```python
from build123d import *

# Parameters (mm, degrees)
SKETCH1_W           = 144
SKETCH1_H           = 50
SKETCH1_R           = 6
BOSS_EXTRUDE1_DEPTH = 37.5
SKETCH2_W           = 51
SKETCH2_H           = 38
CUT_EXTRUDE1_DEPTH  = 157.978501713
CUT_EXTRUDE2_DEPTH  = 116.364639296


with BuildPart() as part:
    # Sketch1 → Boss-Extrude1 (new, symmetric)
    with BuildSketch(Plane(origin=(0, 0, 0), x_dir=(0, 0, -1), z_dir=(1, 0, 0))):
        with Locations((0, 25)):
            Rectangle(SKETCH1_W, SKETCH1_H)
        with Locations((-19, 31)):
            Circle(SKETCH1_R, mode=Mode.SUBTRACT)
        with Locations(Location((19, 31, 0), (0, 0, 180))):
            Circle(SKETCH1_R, mode=Mode.SUBTRACT)
    extrude(amount=BOSS_EXTRUDE1_DEPTH, both=True)

    # Sketch2 → Cut-Extrude1 (cut, through all)
    with BuildSketch(Plane.XY.offset(72)):
        with Locations((0, 31)):
            Rectangle(SKETCH2_W, SKETCH2_H)
    extrude(amount=-CUT_EXTRUDE1_DEPTH, mode=Mode.SUBTRACT)

    # Sketch3 → Cut-Extrude2 (cut, through all)
    with BuildSketch(Plane(origin=(37.5, 0, 0), x_dir=(0, 0, -1), z_dir=(1, 0, 0))):
        with BuildLine():
            Line((72, 12), (72, 50))
            Line((72, 50), (37.5, 50))
            ThreePointArc((37.5, 50), (49.502162082, 26.235515574), (72, 12))
        make_face()
        with BuildLine():
            Line((-72, 50), (-37.5, 50))
            ThreePointArc((-37.5, 50), (-49.502162082, 26.235515574), (-72, 12))
            Line((-72, 12), (-72, 50))
        make_face()
    extrude(amount=-CUT_EXTRUDE2_DEPTH, mode=Mode.SUBTRACT)


solid = part.part
```
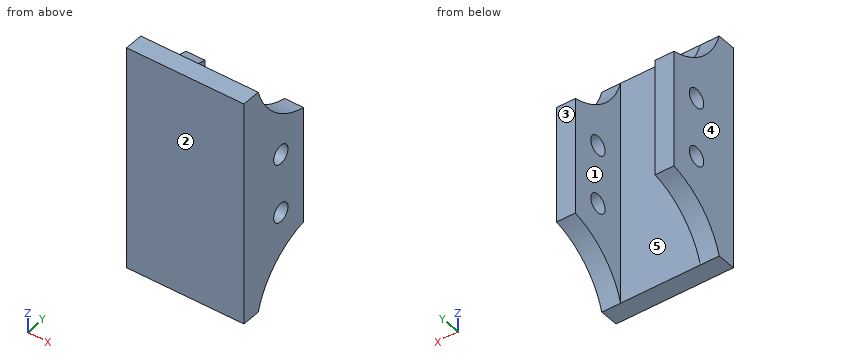
Build history of the part. All positions in model axes, mm. Face numbers are marked on the shaded views. A direction names the side the tool comes from. Give positions to 0.01 mm unless a question says otherwise; leave off trailing zeros. Order: outer loops, then holes, each group sorted by start corner. A loop starts at its lowest first (then second) coordinate and runs counter-clockwise, first axis right, second up. Notation, with made-up numbers: M -39,29.5 L -28,29.5 A24 ccw -28,49.5 Z; hole C 28.5,12 d6. An arc over 180 degrees is marked long. Write item = value, one per line. Start each with the question number.
(1) Two-plate mould, pull along X, no slides. Class the marked faces 3, 4 and 5: released by +X, released by -X, zero draft, split by the parting line, or undercut.
(2) Slice it at A-A on z = 19. Write the cut outline in (x, y), plus the area to 3 significant figures.
(3) Pin check, flat tips, straight feed: pin 1 Ø15.5 at (x, z) = (11, -3.5) entering from +Y; pin 2 Ø14 at (y, z) = (31, 19) entering from -X; pin 3 Ø10 at (x, y) = (-30, 21) entering from -Z. Stop position of each tip, or through.
(4) Slice it at D-D on y = 31. Write the cut outline in (x, z).
(5) Which spindle directions (+Z, -Z, +X, -X, +Y, -Y) get a long thin tool onto all of the face, cutting with end or side? Do the marked faces 1 and 2. Say none if no direction does.
(6) Slice it at C-C on z = 0. Write the cut outline in (x, y), plus the area to 3 significant figures.
(7) Slice it at B-B on y = 38.5. Write the cut outline in (x, z), plus the area to 3 significant figures.
(8) Probe L1, parallel to X at y = 14, z = 21; L2, parallel to Z at x = 35.25, y = 31; L3, parallel to Y at x = -28, z = -19. List the from-to ranges inside material, lowest first. Write a range as [from, to].
Responses:
q1.face_3 = zero draft
q1.face_4 = released by -X
q1.face_5 = undercut
q2.outline = M -37.5,0 L 37.5,0 L 37.5,25 L 25.5,25 L 25.5,12 L -25.5,12 L -25.5,25 L -37.5,25 Z; M -37.5,37 L -25.5,37 L -25.5,50 L -37.5,50 Z; M 25.5,37 L 37.5,37 L 37.5,50 L 25.5,50 Z
q2.area = 1,520 mm2
q3.pin_1 = 12
q3.pin_2 = -37.5
q3.pin_3 = -62.49
q4.outline = M -37.5,-45.68 L -25.5,-45.68 L -25.5,-25 L -37.5,-25 Z; M -37.5,-13 L -25.5,-13 L -25.5,13 L -37.5,13 Z; M -37.5,25 L -25.5,25 L -25.5,45.68 L -37.5,45.68 Z; M 25.5,-45.68 L 37.5,-45.68 L 37.5,-25 L 25.5,-25 Z; M 25.5,-13 L 37.5,-13 L 37.5,13 L 25.5,13 Z; M 25.5,25 L 37.5,25 L 37.5,45.68 L 25.5,45.68 Z
q5.face_1 = +Z, -Z, +Y
q5.face_2 = +Z, -Z, +X, -X, -Y
q6.outline = M -37.5,0 L 37.5,0 L 37.5,50 L 25.5,50 L 25.5,12 L -25.5,12 L -25.5,50 L -37.5,50 Z
q6.area = 1,810 mm2
q7.outline = M -37.5,-41.31 L -25.5,-41.31 L -25.5,41.31 L -37.5,41.31 Z; M 25.5,-41.31 L 37.5,-41.31 L 37.5,41.31 L 25.5,41.31 Z
q7.area = 1,980 mm2
q8.L1 = [-37.5, -25.5], [25.5, 37.5]
q8.L2 = [-45.68, -25], [-13, 13], [25, 45.68]
q8.L3 = [0, 25], [37, 50]
